Input: dimensioned drawing with shaded views. Units: mm. Origin: part minimum x, y, z. A direction names the side the tool comes from. Round coordinates to 2 decimals unless told otherwise and drop trailing zeros. Order: outer loops, then holes, each group sorted by start corner. A loop starts at its lowest first (then second) coordinate and runs counter-clockwise, first axis right, second up. Notation, with made-up numbers: (-26, -18.5) - (-16, -18.5) arc R10 cw to (-16, 0.5) - close; hole circle Ø2 at (-19, 66.25). An arc over 180 degrees is marked (long way). Return JSON: item names as keys, results as strings. Group by question number.
1) Section B-B, the plane z = 16. Return loops of the section in (x, y).
2) Contact query for flat-ended pins moving along their axis: P1, Ø3.5, axis at x = 16, z = 27.95, coming from the -Y side; P2, Ø4, axis at x = 8, y = 3, coming from the -Z side; P3, Ø5, axis at y = 8, z = 12, coming from the -X side. Output: stop coordinate, or through.
3) Section D-D, the plane z = 4.05. Return loops of the section in (x, y).
4) Ray query, line 1 (Z direction, x = 16, y = 3.25); line 2 (Z direction, x = 27.95, y = 2.2); line 3 (X direction, y = 10.5, z = 13.5). Return the intervals inside material, ascending. Write a range as from..to.
5) Mould query, pull axis Z, two halves, no side actions, for the marked faces 3, 4 and 5. Classes: pulls with the +Z half, pulls with the -Z half, needs draft (parallel to the pull), parting line crosses it, or undercut.
6) Section A-A, the plane x = 16. Return loops of the section in (y, z).
7) Section C-C, the plane x = 27.95. Return loops of the section in (y, z).
8) Access query for the marked faces 1 and 2. Directions: +Z, -Z, +X, -X, +Y, -Y. A direction counts if a zero-diameter tool reaches every point of the face in a straight line with its end or side. Return the directions, or none.
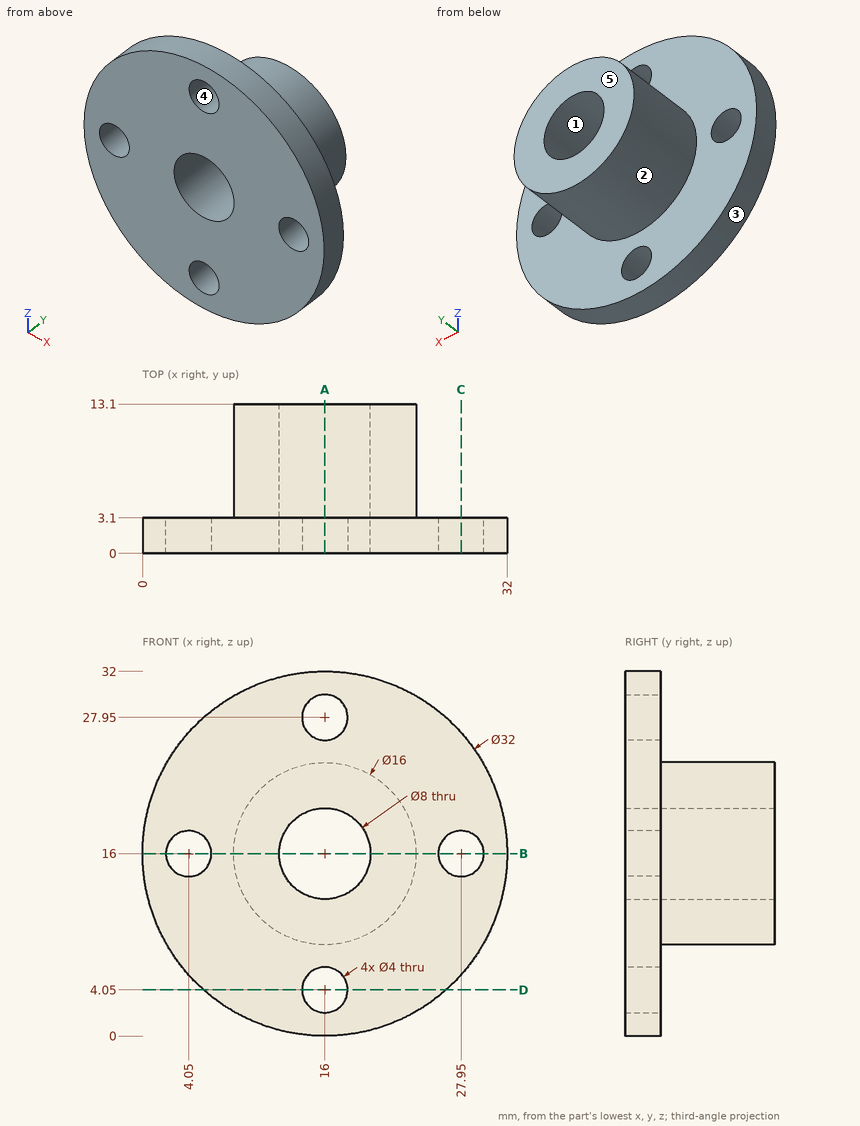
Geometry check:
{
 "1": {"outline": "(0, 0) - (2.05, 0) - (2.05, 3.1) - (0, 3.1) - close; (6.05, 0) - (12, 0) - (12, 13.1) - (8, 13.1) - (8, 3.1) - (6.05, 3.1) - close; (20, 0) - (25.95, 0) - (25.95, 3.1) - (24, 3.1) - (24, 13.1) - (20, 13.1) - close; (29.95, 0) - (32, 0) - (32, 3.1) - (29.95, 3.1) - close"},
 "2": {"P1": "through", "P2": "z = 1.17", "P3": "x = 8.14"},
 "3": {"outline": "(5.36, 0) - (14, 0) - (14, 3.1) - (5.36, 3.1) - close; (18, 0) - (26.64, 0) - (26.64, 3.1) - (18, 3.1) - close"},
 "4": {"line 1": "8..12, 20..24", "line 2": "5.36..14, 18..26.64", "line 3": "8.4..12.88, 19.12..23.6"},
 "5": {"face 3": "parting line crosses it", "face 4": "undercut", "face 5": "needs draft"},
 "6": {"outline": "(0, 0) - (3.1, 0) - (3.1, 2.05) - (0, 2.05) - close; (0, 6.05) - (3.1, 6.05) - (3.1, 8) - (13.1, 8) - (13.1, 12) - (0, 12) - close; (0, 20) - (13.1, 20) - (13.1, 24) - (3.1, 24) - (3.1, 25.95) - (0, 25.95) - close; (0, 29.95) - (3.1, 29.95) - (3.1, 32) - (0, 32) - close"},
 "7": {"outline": "(0, 5.36) - (3.1, 5.36) - (3.1, 14) - (0, 14) - close; (0, 18) - (3.1, 18) - (3.1, 26.64) - (0, 26.64) - close"},
 "8": {"face 1": "+Y, -Y", "face 2": "+Y"}
}
